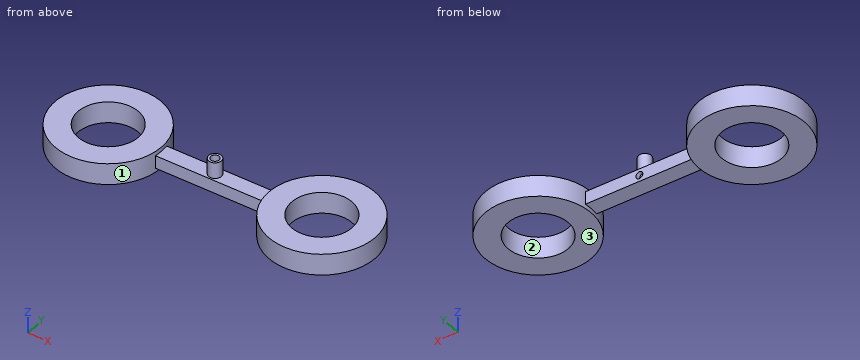
from build123d import *

# Parameters (mm, degrees)
CYLINDER136_R     = 0.2
CYLINDER136_DEPTH = 9
CYLINDER_R        = 1.422
CYLINDER_DEPTH    = 2
CYLINDER139_R     = 1.422
CYLINDER139_DEPTH = 2
CYLINDER138_R     = 0.165
CYLINDER138_DEPTH = 8
CYLINDER142_R     = 2.5
CYLINDER142_DEPTH = 1
CYLINDER141_R     = 2.5
CYLINDER141_DEPTH = 1
CYLINDER140_R     = 0.3
CYLINDER140_DEPTH = 0.75
BOX_W             = 10
BOX_H             = 0.75
BOX_DEPTH         = 0.6


with BuildPart() as bowtienozzle:
    # Cylinder136 → Cylinder136 (new body)
    with BuildSketch(Plane.XY):
        Circle(CYLINDER136_R)
    extrude(amount=CYLINDER136_DEPTH)


with BuildPart() as mountinghole1:
    # Cylinder → Cylinder (new body)
    with BuildSketch(Plane(origin=(-5, 0, -1), x_dir=(1, 0, 0), z_dir=(0, 0, 1))):
        Circle(CYLINDER_R)
    extrude(amount=CYLINDER_DEPTH)


with BuildPart() as mountinghole2:
    # Cylinder139 → Cylinder139 (new body)
    with BuildSketch(Plane(origin=(5, 0, -1), x_dir=(1, 0, 0), z_dir=(0, 0, 1))):
        Circle(CYLINDER139_R)
    extrude(amount=CYLINDER139_DEPTH)


with BuildPart() as fusion001:
    # Cylinder138 → Cylinder138 (new body)
    with BuildSketch(Plane(origin=(0, 0, 0), x_dir=(1, 0, 0), z_dir=(0, 1, 0))):
        Circle(CYLINDER138_R)
    extrude(amount=CYLINDER138_DEPTH)

    # Fusion001: union BowTieNozzle, MountingHole1, MountingHole2
    add(bowtienozzle.part)
    add(mountinghole1.part)
    add(mountinghole2.part)


with BuildPart() as obj1:
    # Cylinder142 → Cylinder142 (new body)
    with BuildSketch(Plane(origin=(5, 0, -0.5), x_dir=(1, 0, 0), z_dir=(0, 0, 1))):
        Circle(CYLINDER142_R)
    extrude(amount=CYLINDER142_DEPTH)


with BuildPart() as obj2:
    # Cylinder141 → Cylinder141 (new body)
    with BuildSketch(Plane(origin=(-5, 0, -0.5), x_dir=(1, 0, 0), z_dir=(0, 0, 1))):
        Circle(CYLINDER141_R)
    extrude(amount=CYLINDER141_DEPTH)


with BuildPart() as nozzle_od:
    # Cylinder140 → Cylinder140 (new body)
    with BuildSketch(Plane.XY.offset(0.3)):
        Circle(CYLINDER140_R)
    extrude(amount=CYLINDER140_DEPTH)


with BuildPart() as cut:
    # Box → Box (new body)
    with BuildSketch(Plane(origin=(-5, -0.375, -0.3), x_dir=(1, 0, 0), z_dir=(0, 0, 1))):
        with Locations((5, 0.375)):
            Rectangle(BOX_W, BOX_H)
    extrude(amount=BOX_DEPTH)

    # Fusion: union obj1, obj2, Nozzle_OD
    add(obj1.part)
    add(obj2.part)
    add(nozzle_od.part)

    # Cut: cut Fusion001
    add(fusion001.part, mode=Mode.SUBTRACT)


solid = cut.part
Can you work these out from the model? Positions are in its coordinate system, mm. Face numbers are marked on the shaded views. Coordinates: 2 decimals unless noted, no trailing zeros. Loops run counter-clockwise (first coordinate to the right, second up) from the corner with the lowest first, then second, coordinate; pieces in that order, holes last. Notation, with made-up numbers: (70, 44) - (79, 44) arc R23 ccw to (79, 83) - close; hole circle Ø5 at (21.25, 50.25). An arc over 180 degrees is marked (long way). Answer as a JSON object with one key per item and string values. Group by question number.
Item 1: If we section it at B-B (x = 0): List the corners of the cut face in (y, z) for me (3 decimals).
Item 2: If we section it at A-A (y = -2): List the corners of the cut face in (x, z) for me, plus the area to 3 significant figures.
Item 3: If we section it at D-D (x = 5): List the corners of the cut face in (y, z) for me, plus the area to 3 significant figures.
Item 4: For pin 1 (2.5 mm diameter, centred on x = 5, y = 0, fed in from -Z); pin 2 (0.5 mm diameter, centred on x = 1, z = 0, fed in from +Y) (3 decimals); pin 3 (2 mm diameter, centred on x = -1, y = 0.5, fed in from +Z), each with a flat end and sliding along its axis, tell me the tip position at first contact or that it passes through.
Item 5: If we section it at C-C (y = 1.05): List the corners of the cut face in (x, z) for me.
Item 6: If we mould it in two halves opening along Y, with no side actions, what happens to the marked faces 1, 2 and 3? For each: released by +Y, released by -Y, zero draft, split by the parting line, or undercut.
Item 7: If I drill on L1, parallel to Y at x = -5, z = 0.1; L2, parallel to X at y = -1.3, z = 0.25; L3, parallel to X at y = 0.5, z = 0.05, over which ranges is the centre line in solid material (lowest first)? Write a range as from..to.
Returned:
{
 "1": {"outline": "(-0.375, -0.3) - (0.375, -0.3) - (0.375, -0.165) - (0, -0.165) - (0, 0) - (-0.2, 0) - (-0.2, 1.05) - (-0.3, 1.05) - (-0.3, 0.3) - (-0.375, 0.3) - close; (0.2, 0.165) - (0.375, 0.165) - (0.375, 0.3) - (0.3, 0.3) - (0.3, 1.05) - (0.2, 1.05) - close"},
 "2": {"outline": "(-6.5, -0.5) - (-3.5, -0.5) - (-3.5, 0.5) - (-6.5, 0.5) - close; (3.5, -0.5) - (6.5, -0.5) - (6.5, 0.5) - (3.5, 0.5) - close", "area": "6.00 mm²"},
 "3": {"outline": "(-2.5, -0.5) - (-1.42, -0.5) - (-1.42, 0.5) - (-2.5, 0.5) - close; (1.42, -0.5) - (2.5, -0.5) - (2.5, 0.5) - (1.42, 0.5) - close", "area": "2.16 mm²"},
 "4": {"pin 1": "passes through", "pin 2": "stops at y = 0.375", "pin 3": "stops at z = 1.05"},
 "5": {"outline": "(-7.27, -0.5) - (-5.96, -0.5) - (-5.96, 0.5) - (-7.27, 0.5) - close; (-4.04, -0.5) - (-2.73, -0.5) - (-2.73, 0.5) - (-4.04, 0.5) - close; (2.73, -0.5) - (4.04, -0.5) - (4.04, 0.5) - (2.73, 0.5) - close; (5.96, -0.5) - (7.27, -0.5) - (7.27, 0.5) - (5.96, 0.5) - close"},
 "6": {"face 1": "split by the parting line", "face 2": "undercut", "face 3": "zero draft"},
 "7": {"L1": "y = -2.5..-1.42, 1.42..2.5", "L2": "x = -7.14..-5.58, -4.42..-2.86, 2.86..4.42, 5.58..7.14", "L3": "x = -7.45..-6.33, -3.67..-2.55, 2.55..3.67, 6.33..7.45"}
}
